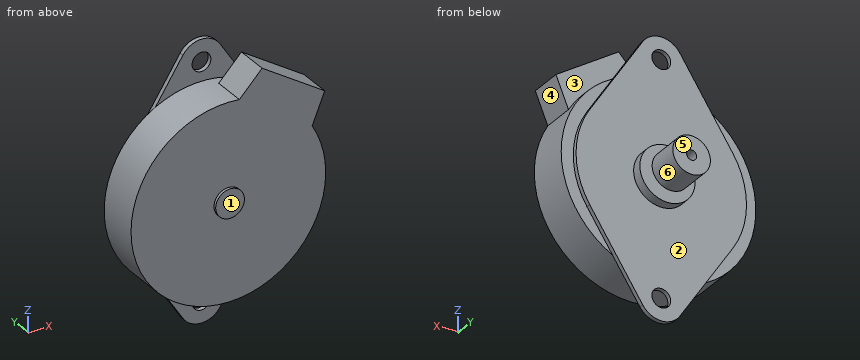
from build123d import *

# Parameters (mm, degrees)
SCHIZZO1_R                   = 17.6
ESTRUSIONE_ESTRUSIONE1_DEPTH = 7.8
SCHIZZO2_R                   = 1.7
ESTRUSIONE_ESTRUSIONE2_DEPTH = 0.8
SCHIZZO3_R                   = 5
ESTRUSIONE_ESTRUSIONE3_DEPTH = 1.8
SCHIZZO4_R                   = 0.9
ESTRUSIONE_ESTRUSIONE4_DEPTH = 5
SCHIZZO5_R                   = 2.6
ESTRUSIONE_ESTRUSIONE5_DEPTH = 0.5
ESTRUSIONE_ESTRUSIONE6_DEPTH = 6
EXTRUDE_START                = 1
SKETCH_1_R                   = 3.4
SKETCH_1_R_2                 = 0.9
EXTRUDE_1_DEPTH              = 6


with BuildPart() as part:
    # Schizzo1 → Estrusione-Estrusione1 (new body)
    with BuildSketch(Plane(origin=(0, 0, 0), x_dir=(1, 0, 0), z_dir=(0, 1, 0))):
        Circle(SCHIZZO1_R)
    extrude(amount=ESTRUSIONE_ESTRUSIONE1_DEPTH)

    # Schizzo2 → Estrusione-Estrusione2 (add)
    with BuildSketch(Plane(origin=(0, 7.8, 0), x_dir=(1, 0, 0), z_dir=(0, 1, 0))):
        with BuildLine():
            Line((-3.357806699, -23.173737374), (-12.937730964, -8.375475972))
            ThreePointArc((-12.937730964, -8.375475972), (-15.412121212, 0), (-12.937730964, 8.375475972))
            Line((-12.937730964, 8.375475972), (-3.357806699, 23.173737374))
            ThreePointArc((-3.357806699, 23.173737374), (0, 25), (3.357806699, 23.173737374))
            Line((3.357806699, 23.173737374), (12.937730964, 8.375475972))
            ThreePointArc((12.937730964, 8.375475972), (15.412121212, 0), (12.937730964, -8.375475972))
            Line((12.937730964, -8.375475972), (3.357806699, -23.173737374))
            ThreePointArc((3.357806699, -23.173737374), (0, -25), (-3.357806699, -23.173737374))
        make_face()
        with Locations((0, 21)):
            Circle(SCHIZZO2_R, mode=Mode.SUBTRACT)
        with Locations((0, -21)):
            Circle(SCHIZZO2_R, mode=Mode.SUBTRACT)
    extrude(amount=ESTRUSIONE_ESTRUSIONE2_DEPTH)

    # Schizzo3 → Estrusione-Estrusione3 (add)
    with BuildSketch(Plane(origin=(0, 8.6, 0), x_dir=(1, 0, 0), z_dir=(0, 1, 0))):
        Circle(SCHIZZO3_R)
    extrude(amount=ESTRUSIONE_ESTRUSIONE3_DEPTH)

    # Schizzo4 → Estrusione-Estrusione4 (add)
    with BuildSketch(Plane(origin=(0, 10.4, 0), x_dir=(1, 0, 0), z_dir=(0, 1, 0))):
        Circle(SCHIZZO4_R)
    extrude(amount=ESTRUSIONE_ESTRUSIONE4_DEPTH)

    # Schizzo5 → Estrusione-Estrusione5 (add)
    with BuildSketch(Plane.XZ):
        Circle(SCHIZZO5_R)
    extrude(amount=ESTRUSIONE_ESTRUSIONE5_DEPTH)

    # Schizzo6 → Estrusione-Estrusione6 (add)
    with BuildSketch(Plane.XZ):
        with BuildLine():
            Line((6.100676559, 21.792297849), (17.423572743, 14.440969942))
            Line((17.423572743, 14.440969942), (15.161900105, 8.937381339))
            ThreePointArc((15.161900105, 8.937381339), (9.583953419, 14.761701692), (1.993791209, 17.486703423))
            Line((1.993791209, 17.486703423), (6.100676559, 21.792297849))
        make_face()
    extrude(amount=-ESTRUSIONE_ESTRUSIONE6_DEPTH)

    # Эскиз1 → Бобышка-Вытянуть1 (add)
    with BuildSketch(Plane(origin=(0, 10.4, 0), x_dir=(1, 0, 0), z_dir=(0, 1, 0)).offset(EXTRUDE_START)):
        Circle(SKETCH_1_R)
        Circle(SKETCH_1_R_2, mode=Mode.SUBTRACT)
    extrude(amount=EXTRUDE_1_DEPTH)


solid = part.part
The listing builds one solid part. Answer for the finished solid, in the listing's coordinates (mm). Face numbers are marked on the shaded views. A direction names the side the tool comes from. Give positions to 0.01 mm unless a question says otherwise; leave off trailing zeros. Write each loop counter-clockwise with the first axis right and the second up, starting at its lowest first coordinate (ties: lowest second). Pieces come first, ordered by that corner, then holes.
Item 1: Section D-D, the plane x = 4 is taken. Write down the section's boundary in (y, z).
Item 2: Which of the six approach directions +Z, -Z, +X, -X, +Y, -Y give full straight-line access (tool end or side, diameter ignored) to the marked faces 4, 5 and 6?
Item 3: Find the intervals of material crossed by line 1 along Z through (x, y) = (0, 8.1); line 2 along Z through (x, y) = (0, 16.75); line 3 along Y through (x, z) = (-5.5, -16), in increasing order.
Item 4: Flat-ended cylindrical pins translate along their axes: P1, Ø8, axis at y = 5.5, z = -16.5, coming from the +X side; P2, Ø4, axis at x = 6.5, z = 1, coming from the -Y side; P3, Ø10, axis at x = 15, z = 4.5, coming from the +Y side. Find the tip coordinate at first contact, or state that the pin passes through.
Item 5: Determine the mould class of the marked faces 1, 2 and 3 for opening direction Y: released by +Y, released by -Y, zero draft, split by the parting line, or undercut.
Item 6: Section C-C, the plane z = 21 is taken. Write down the section's boundary in (x, y).
Item 7: Section B-B, the plane x = 0 is taken. Count the separate pieces of the cut face and the enclosed holes in it, plus the area to 3 significant figures.
Item 8: Section A-A, the plane z = -21 is taken. Write down the section's boundary in (x, y).
Completed:
1. outline: (0, -17.14) - (7.8, -17.14) - (7.8, -22.18) - (8.6, -22.18) - (8.6, -3) - (10.4, -3) - (10.4, 3) - (8.6, 3) - (8.6, 22.18) - (7.8, 22.18) - (7.8, 17.14) - (6, 17.14) - (6, 19.59) - (0, 19.59) - close
2. face 4: +X, +Y, -Y
2. face 5: +Z, -Z, +X, -X, +Y
2. face 6: +Y
3. line 1: z = -25 to -22.7, -19.3 to 19.3, 22.7 to 25
3. line 2: z = -3.4 to -0.9, 0.9 to 3.4
3. line 3: y = 0 to 8.6
4. P1: stops at x = 12.39
4. P2: stops at y = 0
4. P3: stops at y = 8.6
5. face 1: released by -Y
5. face 2: released by +Y
5. face 3: undercut
6. outline: (-4.77, 7.8) - (-1.7, 7.8) - (-1.7, 8.6) - (-4.77, 8.6) - close; (1.7, 7.8) - (4.77, 7.8) - (4.77, 8.6) - (1.7, 8.6) - close; (5.34, 0) - (7.32, 0) - (7.32, 6) - (5.34, 6) - close
7. separate pieces: 3
7. enclosed holes: 0
7. area: 369 mm2
8. outline: (-4.77, 7.8) - (-1.7, 7.8) - (-1.7, 8.6) - (-4.77, 8.6) - close; (1.7, 7.8) - (4.77, 7.8) - (4.77, 8.6) - (1.7, 8.6) - close
